Here's the drawing with two shaded views (mm, measured from the low corner). I have some questions. A direction names the side the tool comes from. Coordinates: 2 decimals unless noted, no trailing zeros. Write each loop counter-clockwise with the first axis right and the second up, starting at its lowest first coordinate (ties: lowest second). Pieces come first, ordered by that corner, then holes.
Item 1: Which directions (+Z, -Z, +X, -X, +Y, -Y) give clear straight access to the entire face, cutting with the end or side of a thin tool? Please do the marked faces 1, 2 and 3.
Item 2: I want a section at B-B on y = 44. Please give me the cut outline in (x, z), then the cut area to 3 significant figures.
Item 3: I want a section at D-D on x = 27.5. Please give me the cut outline in (y, z).
Item 4: Thinking about a two-plate mould opening in Z: for the marked faces 4, 5 and 6, which applies, +Z half, -Z half, draft (parallel to the pull), parting line (faces both ways), or undercut?
Item 5: If I drill on probe 1 along Z at (x, y) = (15, 57); probe 2 along Z at (x, y) = (17.5, 29); probe 3 along Y at (x, z) = (12, 13.5), over which ranges is the centre line in solid material (lowest first)?
Item 6: I want a section at C-C on z = 1.5. Please give me the cut outline in (x, y), then the cut area to 3 significant figures.
Item 7: For P1, Ø12, axis at x = 12, y = 23.5, coming from the -Z side; P2, Ø8, axis at x = 17.5, y = 35.5, coming from the -Z side; P3, Ø3, axis at x = 21, z = 12.5, coming from the +Y side, each with a flat end and sliding along its axis, tell me the tip position at first contact or that it passes through.
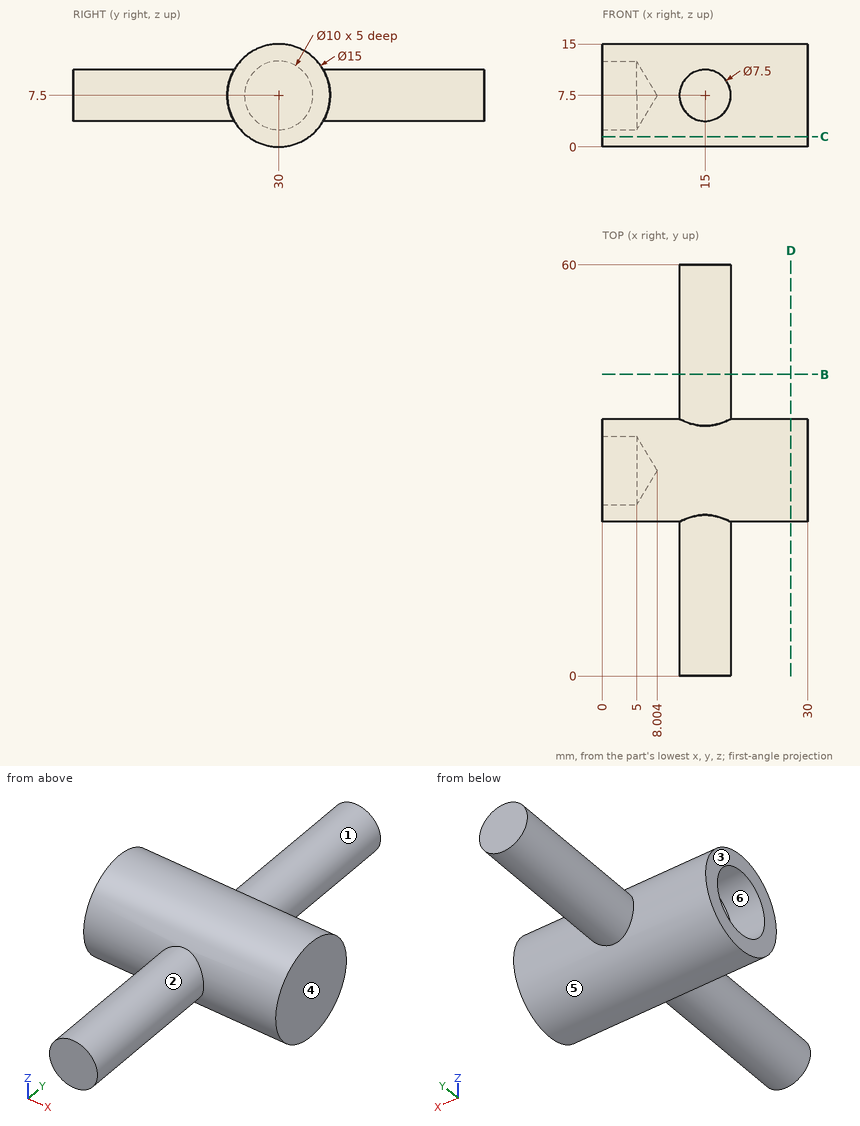
Response values:
1. face 1: +Y
1. face 2: -Y
1. face 3: +Z, -Z, -X, +Y, -Y
2. outline: circle Ø7.5 at (15, 7.5)
2. area: 44.2 mm2
3. outline: circle Ø15 at (30, 7.5)
4. face 4: draft
4. face 5: parting line
4. face 6: undercut
5. probe 1: z = 3.75 to 11.25
5. probe 2: z = 0.07 to 14.93
5. probe 3: y = 25.5 to 34.5
6. outline: (0, 25.5) - (30, 25.5) - (30, 34.5) - (0, 34.5) - close
6. area: 270 mm2
7. P1: stops at z = 0.02
7. P2: stops at z = 0.15
7. P3: stops at y = 36.63
